Verification items for this drawing (mm, ordinates from the low corner). A direction names the side the tool comes from. Give positions to 0.01 mm unless a question says otherwise; leave off trailing zeros. Loops run counter-clockwise (first coordinate to the right, second up) from the corner with the lowest first, then second, coordinate; pieces in that order, holes last. Notation, with made-up numbers: (4, -9) -> (29, -9) arc R9 cw to (29, -2) -> close; hole circle Ø2 at (-27.75, 63.5). An arc over 180 degrees is marked (long way). Use one line per item in the form item = value. Start each with the question number.
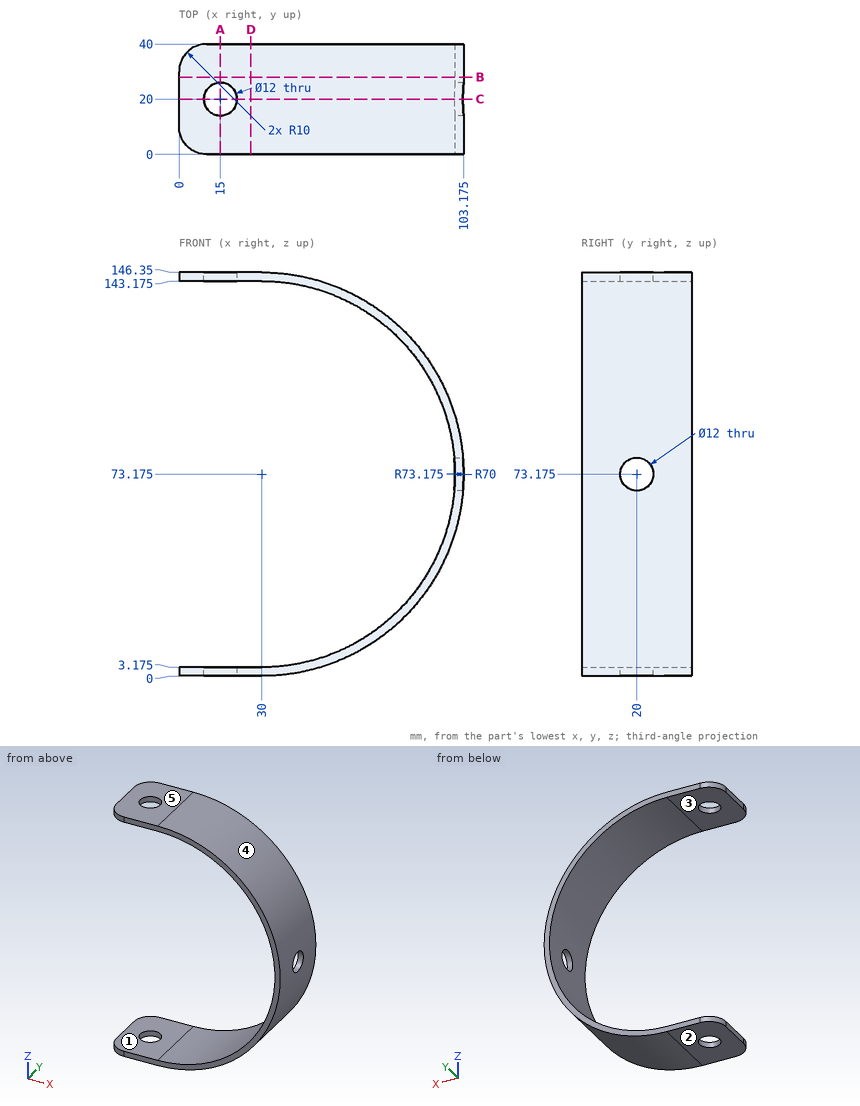
Item 1: Gauge pin test, flat ends, axial feed: pin 1 Ø4 at (y, z) = (34, 107.5) entering from +X; pin 2 Ø6 at (x, y) = (89, 15.5) entering from +Z; pin 3 Ø5 at (y, z) = (29, 43) entering from +X; pin 4 Ø14 at (y, z) = (20, 73.175) entering from +X (3 decimals). Record the tip position at first contact, or that the pin passes through.
Item 2: Tool access check on the marked faces 1 and 2. Record the directions out of +Z, -Z, +X, -X, +Y, -Y that give a thin tool (end or side, any length) a straight path to the whole face; none if there is none.
Item 3: Draft check along Z on the marked faces 3, 4 and 5. Enter one of: +Z half, -Z half, draft (parallel to the pull), parting line (faces both ways), or undercut.
Item 4: Sectioned sample at D-D, the plane x = 26. Enter the section's corners in (y, z) (3 decimals), and give its area (3 significant figures).
Item 5: Sectioned sample at C-C, the plane y = 20. Enter the section's corners in (x, z) (3 decimals), and give its area (3 significant figures).
Item 6: Material ranges on line 1 (Y direction, x = 15, z = 145); line 2 (Z direction, x = 32, y = 29.5); line 3 (Z direction, x = 16, y = 12.5) (3 decimals), recorded low to high.
Item 7: Sectioned sample at A-A, the plane x = 15. Enter the section's corners in (y, z) (3 decimals).
Item 8: Sectioned sample at B-B, the plane y = 28. Enter the section's corners in (x, z) (3 decimals), and give its area (3 significant figures).
Outcome:
q1.pin_1 = 95.65
q1.pin_2 = 120.28
q1.pin_3 = 97.74
q1.pin_4 = 103.175
q2.face_1 = -X, +Y, -Y
q2.face_2 = -Z, +X, -X, +Y, -Y
q3.face_3 = undercut
q3.face_4 = parting line
q3.face_5 = +Z half
q4.outline = (0, 0) -> (40, 0) -> (40, 3.175) -> (0, 3.175) -> close; (0, 143.175) -> (40, 143.175) -> (40, 146.35) -> (0, 146.35) -> close
q4.area = 254 mm^2
q5.outline = (0, 0) -> (9, 0) -> (9, 3.175) -> (0, 3.175) -> close; (0, 143.175) -> (9, 143.175) -> (9, 146.35) -> (0, 146.35) -> close; (21, 0) -> (30, 0) arc R73.175 ccw to (102.929, 67.175) -> (99.742, 67.175) arc R70 cw to (30, 3.175) -> (21, 3.175) -> close; (21, 143.175) -> (30, 143.175) arc R70 cw to (99.742, 79.175) -> (102.929, 79.175) arc R73.175 ccw to (30, 146.35) -> (21, 146.35) -> close
q5.area = 790 mm^2
q6.line_1 = 0 to 14, 26 to 40
q6.line_2 = 0.03 to 3.2, 143.15 to 146.32
q6.line_3 = 0 to 3.175, 143.175 to 146.35
q7.outline = (0, 0) -> (14, 0) -> (14, 3.175) -> (0, 3.175) -> close; (0, 143.175) -> (14, 143.175) -> (14, 146.35) -> (0, 146.35) -> close; (26, 0) -> (40, 0) -> (40, 3.175) -> (26, 3.175) -> close; (26, 143.175) -> (40, 143.175) -> (40, 146.35) -> (26, 146.35) -> close
q8.outline = (0, 0) -> (30, 0) arc R73.175 ccw to (30, 146.35) -> (0, 146.35) -> (0, 143.175) -> (30, 143.175) arc R70 cw to (30, 3.175) -> (0, 3.175) -> close
q8.area = 905 mm^2
